Design review of the part shown in the three views and the two pictorial views. Dimensions are in mm from the part's minimum x, y and z. A direction names the side the tool comes from. Round coordinates to 2 decimals unless told otherwise and drop trailing zeros. Loops run counter-clockwise (first coordinate to the right, second up) from the corner with the lowest first, then second, coordinate; pieces in that order, holes last. Notation, with made-up numbers: (-36.5, -17.75) -> (22.5, -17.75) arc R26 ccw to (22.5, -3.75) -> close; hole circle Ø1 at (-34, 45). An arc over 180 degrees is marked (long way). Use a Markdown table: item, result. Add a question column.
1) Mouldability with a two-part tool opening along X and no side actions: class the marked faces 1, 2, 3 and 4 as released by +X, released by -X, zero draft, split by the parting line, or undercut.
2) For the marked faces 5 and 6, list the 3-axis set-ups (+Z, -Z, +X, -X, +Y, -Y) from which the entire face can be reached by the end or side of a thin tool; tool diameter is ignored.
3) Consider section B-B on z = 11. Give the boundary of the cut face in (x, y).
4) Insertion check: pin 1 (3 mm diameter, centred on x = 12, y = 10, fed in from +Z); pin 2 (3 mm diameter, centred on x = 8.5, z = 11.5, fed in from +Y); pin 3 (8 mm diameter, centred on y = 18, z = 16, fed in from -X). Each pin has a flat end and moves straight along its axis. Give the tip position at first contact, or say it passes through.
5) Wall thickness on probe 1 along X at (y, z) = (10.5, 19.5); probe 2 along Y at (x, z) = (12.25, 8.75); probe 3 along Y at (x, z) = (8, 7.5) (1 decimal): over which ranges is each line inside the solid? List them lowest first.
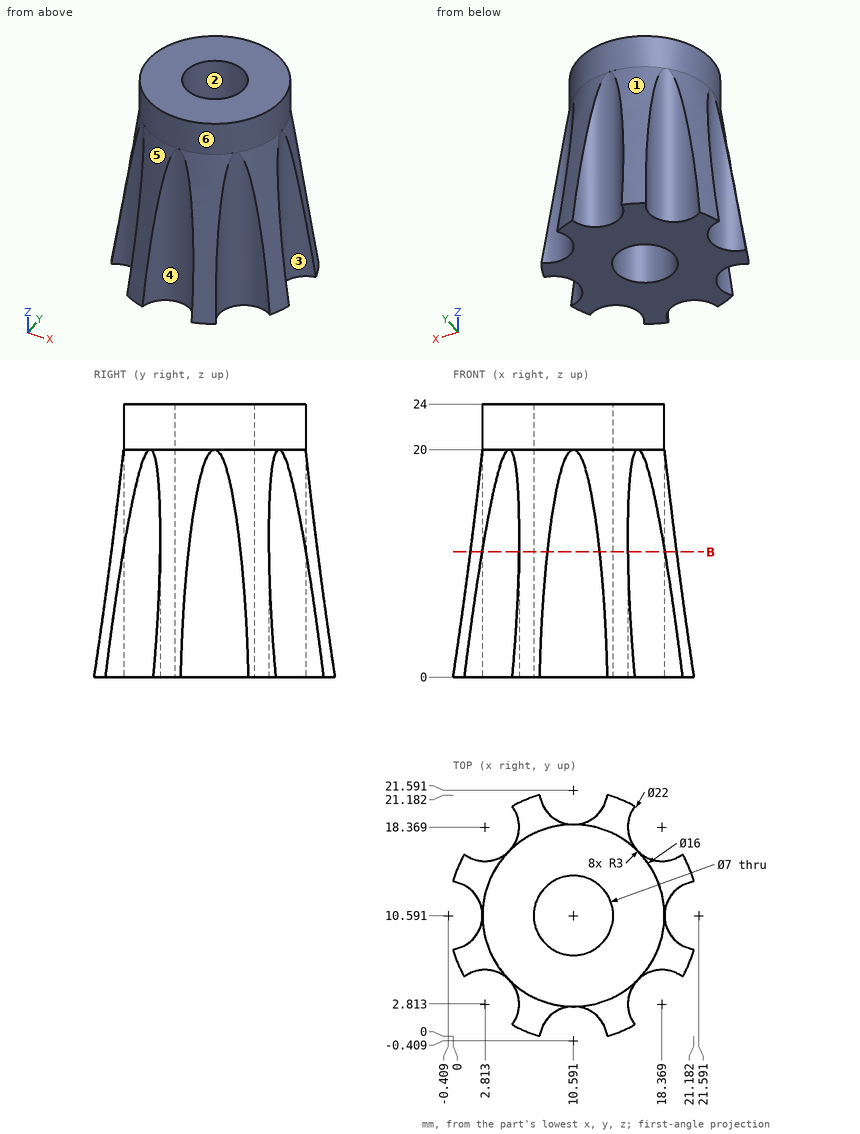
Result set:
| question | item | result |
|---|---|---|
| 1 | face 1 | released by -X |
| 1 | face 2 | undercut |
| 1 | face 3 | released by +X |
| 1 | face 4 | undercut |
| 2 | face 5 | +Z, -X, -Y |
| 2 | face 6 | +Z |
| 3 | outline | (1.53, 8.3) arc R9.35 ccw to (2.56, 5.8) arc R3 cw to (5.8, 2.56) arc R9.35 ccw to (8.3, 1.53) arc R3 cw to (12.88, 1.53) arc R9.35 ccw to (15.38, 2.56) arc R3 cw to (18.62, 5.8) arc R9.35 ccw to (19.66, 8.3) arc R3 cw to (19.66, 12.88) arc R9.35 ccw to (18.62, 15.38) arc R3 cw to (15.38, 18.62) arc R9.35 ccw to (12.88, 19.66) arc R3 cw to (8.3, 19.66) arc R9.35 ccw to (5.8, 18.62) arc R3 cw to (2.56, 15.38) arc R9.35 ccw to (1.53, 12.88) arc R3 cw to start; hole circle Ø7 at (10.59, 10.59) |
| 4 | pin 1 | through |
| 4 | pin 2 | y = 19.78 |
| 4 | pin 3 | x = 2.58 |
| 5 | probe 1 | 2.59 to 7.09, 14.09 to 18.59 |
| 5 | probe 2 | 2.09 to 7.51, 13.67 to 19.09 |
| 5 | probe 3 | 1.1 to 8.2, 12.9 to 20.1 |
